from build123d import *

# Parameters (mm, degrees)
F1_DEPTH = 25
F2_R     = 2.4771890227
F2_R_2   = 2.250855145
F3_DEPTH = 5
F5_DEPTH = 6
F6_R     = 2.5
F7_DEPTH = 25


with BuildPart() as f1:
    # F0 (on Front) → F1 (new body)
    with BuildSketch(Plane.XZ):
        with BuildLine():
            Line((-6.5901947265, 0), (0, 0))
            Line((0, 0), (0, 1.4541312475))
            Line((0, 1.4541312475), (0, 1.9))
            Line((0, 1.9), (-2.1543446928, 1.9))
            Line((-2.1543446928, 1.9), (-4.3302040632, 1.9))
            ThreePointArc((-4.3302040632, 1.9), (-4.4665240815, 2.2584645112), (-4.5287162974, 2.6368982326))
            Line((-4.5287162974, 2.6368982326), (-3.7099796114, 3.4556349186))
            Line((-3.7099796114, 3.4556349186), (11.8111070049, 18.9767215349))
            Line((11.8111070049, 18.9767215349), (13.9676899182, 21.1333044483))
            Line((13.9676899182, 21.1333044483), (12.624187034, 22.4768073325))
            Line((12.624187034, 22.4768073325), (-7.1773967105, 2.6752235881))
            Line((-7.1773967105, 2.6752235881), (-7.4079630013, 2.4446572973))
            ThreePointArc((-7.4079630013, 2.4446572973), (-7.6680055311, 0.9985643577), (-6.5901947265, 0))
        make_face()
        with BuildLine():
            Line((0, 1.4541312475), (0, 0))
            Line((0, 0), (50, 0))
            Line((50, 0), (50, 1.9))
            Line((50, 1.9), (0.0456553072, 1.9))
            ThreePointArc((0.0456553072, 1.9), (0.0342117177, 1.6758999378), (0, 1.4541312475))
        make_face()
    extrude(amount=F1_DEPTH)

    # F2 (on face) → F3 (cut)
    with BuildSketch(Plane(origin=(-4.9263101493, 0, 4.9263101493), x_dir=(0, -1, 0), z_dir=(-0.7071067812, 0, 0.7071067812))):
        with Locations((18.7418013811, 17.0671120286)):
            Circle(F2_R)
        with Locations((6.0519576073, 16.9952586293)):
            Circle(F2_R_2)
    extrude(amount=-F3_DEPTH, mode=Mode.SUBTRACT)

    # F4 (on face) → F5 (cut)
    with BuildSketch(Plane(origin=(-4.9263101493, 0, 4.9263101493), x_dir=(0, -1, 0), z_dir=(-0.7071067812, 0, 0.7071067812))):
        with BuildLine():
            Line((0, 24.8201511429), (0, 22.8517428041))
            ThreePointArc((0, 22.8517428041), (0.6533469706, 24.2230461475), (2.0500576593, 24.8201511429))
            Line((2.0500576593, 24.8201511429), (0, 24.8201511429))
        make_face()
        with BuildLine():
            ThreePointArc((22.6727053523, 24.8201511429), (24.2438861053, 24.062743833), (25, 22.4909402288))
            Line((25, 22.4909402288), (25, 24.8201511429))
            Line((25, 24.8201511429), (22.6727053523, 24.8201511429))
        make_face()
    extrude(amount=-F5_DEPTH, mode=Mode.SUBTRACT)

    # F6 (on face) → F7 (cut)
    with BuildSketch(Plane.XY.offset(1.9)):
        with BuildLine():
            ThreePointArc((45.8127014494, 0), (48.6544638234, -1.190988554), (50, -3.9629192031))
            Line((50, -3.9629192031), (50, 0))
            Line((50, 0), (45.8127014494, 0))
        make_face()
        with BuildLine():
            ThreePointArc((50, -20.6832401454), (48.5516700012, -23.6773197936), (45.5, -25))
            Line((45.5, -25), (50, -25))
            Line((50, -25), (50, -20.6832401454))
        make_face()
        with BuildLine():
            Line((33, -15), (43, -15))
            ThreePointArc((43, -15), (45.5, -12.5), (43, -10))
            Line((43, -10), (33, -10))
            ThreePointArc((33, -10), (30.5, -12.5), (33, -15))
        make_face()
        with Locations((18, -12.5)):
            Circle(F6_R)
    extrude(amount=-F7_DEPTH, mode=Mode.SUBTRACT)


solid = f1.part
Model file for the job. Use its own axes, mm. A direction names the side the tool comes from. Coordinates: 2 decimals unless noted, no trailing zeros. Loops run counter-clockwise (first coordinate to the right, second up) from the corner with the lowest first, then second, coordinate; pieces in that order, holes last. Notation, with made-up numbers: (-13, -24) -> (43, -24) arc R24 ccw to (43, -3) -> close; hole circle Ø5 at (57.25, -26). An arc over 180 degrees is marked (long way). Use one line per item in the form item = value. Start each with the question number.
(1) Cut at D-D on y = -22. Give the cut face in (x, z).
(2) Cut at C-C on y = -18. Give the cut face in (x, z), and give its area (3 significant figures).
(3) Flat gauge pins, fed straight in: pin 1 (2 mm diameter, centred on y = -18.5, z = 4, fed in from -X); pin 2 (1.5 mm diameter, centred on x = 2.5, y = -18, fed in from +Z); pin 3 (5 mm diameter, centred on y = -9, z = 17, fed in from -X). Where does each tip first touch, or does it go through?
(4) Tool access for faces 1 (the flat face through (38, -10, 1)), 2 (the flat face through (-2, -12, 1.9)), 3 (the cylindrical face through (12.76, -24.23, 21.29)): list every direction of +Z, -Z, +X, -X, +Y, -Y with a clear straight run to the whole face (end or side of a thin tool).
(5) Pull direction Y, two halves, no side cores. Call faces 4 (the cylindrical face through (48.59, -23.64, 0.96)), 5 (the cylindrical face through (30.5, -12.4, 1)), 6 (the flat face through (25, -12, 1.9)): pulls with the +Y half, pulls with the -Y half, needs draft (parallel to the pull), parting line crosses it, or undercut.
(6) Probe probe 1 along Y at (x, z) = (18, 1.3); probe 2 along Z at (x, y) = (21, -3.75); probe 3 along Z at (x, y) = (8.5, -7.75). List the from-to ranges inside material, lowest first. Write a range as from..to.
(7) Cut at B-B on x = 18. Give the cut face in (y, z), and give its area (3 significant figures).
(8) Cut at A-A on y = -12.5. Give the cut face in (x, z), and give its area (3 significant figures).
Values:
q1.outline = (-7.41, 2.44) arc R1.53 ccw to (-6.59, 0) -> (49.68, 0) -> (49.68, 1.9) -> (0.05, 1.9) arc R2.2 cw to (0, 1.45) -> (0, 1.9) -> (-4.33, 1.9) arc R1.92 cw to (-4.53, 2.64) -> (13.97, 21.13) -> (12.62, 22.48) -> close
q2.outline = (-7.41, 2.44) arc R1.53 ccw to (-6.59, 0) -> (50, 0) -> (50, 1.9) -> (0.05, 1.9) arc R2.2 cw to (0, 1.45) -> (0, 1.9) -> (-4.33, 1.9) arc R1.92 cw to (-4.53, 2.64) -> (6.81, 13.98) -> (5.47, 15.32) -> close; (8.81, 18.67) -> (10.16, 17.32) -> (13.97, 21.13) -> (12.62, 22.48) -> close
q2.area = 154 mm2
q3.pin_1 = -6.85
q3.pin_2 = 13.1
q3.pin_3 = 4.65
q4.face_1 = +Z, -Z
q4.face_2 = +X, +Y, -Y
q4.face_3 = +Z, +X, -Y
q5.face_4 = pulls with the -Y half
q5.face_5 = undercut
q5.face_6 = needs draft
q6.probe_1 = -25..-15, -10..0
q6.probe_2 = 0..1.9
q6.probe_3 = 0..1.9, 17.62..18.35
q7.outline = (-25, 0) -> (-15, 0) -> (-15, 1.9) -> (-25, 1.9) -> close; (-10, 0) -> (0, 0) -> (0, 1.9) -> (-10, 1.9) -> close
q7.area = 38.0 mm2
q8.outline = (-7.41, 2.44) arc R1.53 ccw to (-6.59, 0) -> (15.5, 0) -> (15.5, 1.9) -> (0.05, 1.9) arc R2.2 cw to (0, 1.45) -> (0, 1.9) -> (-4.33, 1.9) arc R1.92 cw to (-4.53, 2.64) -> (13.97, 21.13) -> (12.62, 22.48) -> close; (20.5, 0) -> (30.5, 0) -> (30.5, 1.9) -> (20.5, 1.9) -> close; (45.5, 0) -> (50, 0) -> (50, 1.9) -> (45.5, 1.9) -> close
q8.area = 125 mm2
